Autodesk Inventor part; units mm, degrees
ref_plane "YZ Plane" through (0, 0, 0) normal (1, 0, 0) x (0, 1, 0)
ref_plane "XZ Plane" through (0, 0, 0) normal (0, 1, 0) x (-1, 0, 0)
ref_plane "XY Plane" through (0, 0, 0) normal (0, 0, 1) x (1, 0, 0)
sketch "Sketch1" plane through (0, 0, 0) normal (0, 0, 1) x (1, 0, 0)
  circle A0 centre (-414.4261, -56.251) radius 4.7625
  point P0 (0, 0)
  dimension "d0" = 9.525
extrude "Extrusion1" add sketch "Sketch1" against normal blind 50.8
sketch "Sketch2" plane through (-414.4261, -56.251, 0) normal (0, 0, 1) x (1, 0, 0)
  circle A0 centre (0, 0) radius 4.7625
  line L0 (-8.2489, 0) -> (-4.1244, 7.1437)
  line L1 (-4.1244, 7.1437) -> (4.1244, 7.1438)
  line L2 (4.1244, 7.1438) -> (8.2489, 0)
  line L3 (8.2489, 0) -> (4.1244, -7.1437)
  line L4 (4.1244, -7.1437) -> (-4.1244, -7.1438)
  line L5 (-4.1244, -7.1438) -> (-8.2489, 0)
  point P0 (414.4261, 56.251)
  dimension "d3" = 14.2875
extrude "Extrusion2" add sketch "Sketch2" along normal blind 3.175 contours A0 | L0 L1 L2 L3 L4 L5
thread "Thread1"
chamfer "Chamfer1" distance 0.508 angle 45 1 edges at (-419.1886, -56.251, -50.8)
properties part number "375 bolt x4" material "Steel"
CAD build for the part. Positions are in the model's coordinates, mm. A direction names the side the tool comes from. Coordinates: 2 decimals unless noted, no trailing zeros. Order: outer loops, then holes, each group sorted by start corner. A loop starts at its lowest first (then second) coordinate and runs counter-clockwise, first axis right, second up. Notation, with made-up numbers: (15.25, 8) - (34.25, 8) arc R18 cw to (34.25, 41) - close; hole circle Ø5 at (60.5, 67). An arc over 180 degrees is marked (long way). Answer in a Markdown table with one row per item.
1. Drill centre lines: L1, parallel to Z at x = -420, y = -58.5 (3 decimals); L2, parallel to X at y = -56.25, z = -36; L3, parallel to X at y = -53.25, z = -11.5. Where is each one in solid material? Low to high. Write a range as from..to.
Answer:
| item | result |
|---|---|
| L1 | 0..3.175 |
| L2 | -419.19..-409.66 |
| L3 | -418.12..-410.73 |
2. Slice it at D-D, the plane z = -36. List the corners of the cut face in (x, y) (1 decimal).
Answer:
| item | result |
|---|---|
| outline | circle Ø9.5 at (-414.4, -56.3) |
3. Flat gauge pins, fed straight in: P1, Ø2, axis at x = -420, y = -58, coming from the -Z side; P2, Ø6, axis at x = -409, z = -18.5, coming from the +Y side; P3, Ø3, axis at y = -58.5, z = -6.5, coming from the +X side. Where does each tip first touch, or does it go through?
Answer:
| item | result |
|---|---|
| P1 | z = 0 |
| P2 | y = -52.15 |
| P3 | x = -409.72 |
4. Slice it at B-B, the plane y = -50.5. List the corners of the cut face in (x, z) (3 decimals).
Answer:
| item | result |
|---|---|
| outline | (-419.355, 0) - (-409.498, 0) - (-409.498, 3.175) - (-419.355, 3.175) - close |
5. 3-axis set-ups, long thin cutter, end or side, ignore diameter. For faces 1 (the face through (-420.584, -59.873, 1.565)), 2 (the face through (-415, -51, 0)): which of +Z, -Z, +X, -X, +Y, -Y reach the whole face in a straight line?
Answer:
| item | result |
|---|---|
| face 1 | +Z, -Z, -X, -Y |
| face 2 | -Z |
6. Slice it at C-C, the plane x = -421.25. List the corners of the cut face in (y, z) (3 decimals).
Answer:
| item | result |
|---|---|
| outline | (-58.719, 0) - (-53.783, 0) - (-53.783, 3.175) - (-58.719, 3.175) - close |
7. Slice it at A-A, the plane z = 0.5. List the corners of the cut face in (x, y) (1 decimal).
Answer:
| item | result |
|---|---|
| outline | (-422.7, -56.3) - (-418.6, -63.4) - (-410.3, -63.4) - (-406.2, -56.3) - (-410.3, -49.1) - (-418.6, -49.1) - close |
